Design review of the part built by this model. Coordinates are the model's own, in mm. A direction names the side the tool comes from. Coordinates: 2 decimals unless noted, no trailing zeros. Write each loop counter-clockwise with the first axis right and the second up, starting at its lowest first coordinate (ties: lowest second). Pieces come first, ordered by that corner, then holes.
Autodesk Inventor part; units mm, degrees
ref_plane "YZ Plane" through (0, 0, 0) normal (1, 0, 0) x (0, 1, 0)
ref_plane "XZ Plane" through (0, 0, 0) normal (0, 1, 0) x (-1, 0, 0)
ref_plane "XY Plane" through (0, 0, 0) normal (0, 0, 1) x (1, 0, 0)
sketch "Sketch1" plane through (0, 0, 0) normal (0, 1, 0) x (-1, 0, 0)
  line L0 (-60, 75) -> (60, 75)
  line L1 (60, -75) -> (-60, -75)
  line L2 (-60, 75) -> (60, -75) construction
  line L3 (60, 75) -> (-60, -75) construction
  line L4 (-60, -75) -> (-60, -55)
  line L5 (-60, -55) -> (-57, -55)
  line L6 (-60, -55) -> (-57, -55)
  line L7 (-57, -55) -> (-57, -42.5)
  line L8 (-57, -42.5) -> (-60, -42.5)
  line L9 (-60, -42.5) -> (-60, -55)
  line L10 (-57, -42.5) -> (-38.1, -42.5)
  line L11 (-38.1, -42.5) -> (-35.1, -42.5)
  line L12 (-35.1, -42.5) -> (-35.1, -55)
  line L13 (-35.1, -55) -> (-38.1, -55)
  line L14 (-38.1, -55) -> (-38.1, -42.5)
  line L15 (0, 75) -> (0, 64.8)
  line L16 (0, 64.8) -> (-33, 64.8)
  line L17 (-33, 64.8) -> (33, 64.8)
  circle A0 centre (-33, 64.8) radius 1.4
  circle A1 centre (33, 64.8) radius 1.4
  line L18 (0, 75) -> (0, 40)
  line L19 (0, 40) -> (-20, 40)
  line L20 (-20, 40) -> (20, 40)
  circle A2 centre (20, 40) radius 1.4
  circle A3 centre (-20, 40) radius 1.4
  line L21 (-60, -75) -> (-60, -5)
  line L22 (-4, -5) -> (4, -5)
  line L23 (-60, 75) -> (-60, 60)
  line L24 (-60, 60) -> (60, 60)
  line L25 (-20, 40) -> (-21.4, 40)
  line L26 (20, 40) -> (21.4, 40)
  line L27 (-30, 40) -> (-30, 10)
  line L28 (-30, 10) -> (-60, 0)
  line L29 (30, 40) -> (30, 10)
  line L30 (30, 10) -> (60, -5)
  line L31 (-30, 40) -> (-30, 48)
  line L32 (-30, 48) -> (-60, 60)
  line L33 (30, 40) -> (30, 48)
  line L34 (30, 48) -> (60, 60)
  line L35 (0, 75) -> (0, -75)
  line L36 (0, -75) -> (-60, -75)
  line L37 (0, 75) -> (-60, 75)
  line L38 (60, -70) -> (60, -55)
  line L39 (60, -55) -> (57, -55)
  line L40 (57, -55) -> (57, -42.5)
  line L41 (57, -42.5) -> (60, -42.5)
  line L42 (60, -42.5) -> (60, -55)
  line L43 (57, -42.5) -> (38.1, -42.5)
  line L44 (38.1, -42.5) -> (35.1, -42.5)
  line L45 (35.1, -42.5) -> (35.1, -55)
  line L46 (35.1, -55) -> (38.1, -55)
  line L47 (38.1, -55) -> (38.1, -42.5)
  line L48 (60, 75) -> (52, 75)
  line L49 (52, 75) -> (52, 70)
  line L50 (52, 70) -> (60, 70)
  line L51 (60, 70) -> (60, 75)
  line L52 (-60, 75) -> (-52, 75)
  line L53 (-52, 75) -> (-52, 70)
  line L54 (-52, 70) -> (-60, 70)
  line L55 (-60, 70) -> (-60, 75)
  line L56 (60, 70) -> (52, 75)
  line L57 (-52, 75) -> (-60, 70)
  line L58 (60, 75) -> (60, 60)
  line L59 (60, -5) -> (60, -70)
  line L60 (-60, -75) -> (-60, 0)
  line L61 (-60, 60) -> (-60, 75)
  line L62 (57, -75) -> (50, -75)
  line L63 (50, -75) -> (50, -70)
  line L64 (50, -70) -> (60, -70)
  line L65 (60, -70) -> (60, -75)
  line L66 (-60, -75) -> (-50, -75)
  line L67 (-50, -75) -> (-50, -70)
  line L68 (-50, -70) -> (-60, -70)
  line L69 (-60, -70) -> (-60, -75)
  line L70 (-60, -70) -> (-50, -75)
  line L71 (60, -70) -> (50, -75)
  line L72 (33, 64.8) -> (33, 62.8)
  line L73 (33, 62.8) -> (-33, 62.8)
  line L74 (-33, 62.8) -> (-33, 64.8)
  line L75 (0, 62.8) -> (10, 62.8)
  line L76 (10, 62.8) -> (-10, 62.8)
  line L77 (-10, 61.05) -> (10, 61.05)
  line L78 (10, 61.05) -> (10, 64.55)
  line L79 (10, 64.55) -> (-10, 64.55)
  line L80 (-10, 64.55) -> (-10, 61.05)
  line L81 (-10, 61.05) -> (10, 64.55) construction
  line L82 (10, 61.05) -> (-10, 64.55) construction
  line L83 (10, 61.05) -> (-10, 61.05)
  line L84 (-10, 61.05) -> (-10, 60)
  line L85 (-10, 60) -> (10, 60)
  line L86 (10, 60) -> (10, 61.05)
  line L87 (30, 48) -> (30, 23)
  line L88 (30, 23) -> (60, -5)
  line L89 (-30, 48) -> (-30, 23)
  line L90 (-30, 23) -> (-60, 0)
  line L91 (60, -75) -> (31, -75)
  line L92 (31, -75) -> (31, -67)
  line L93 (31, -67) -> (60, -67)
  line L94 (60, -67) -> (60, -75)
  line L95 (-60, -75) -> (-31, -75)
  line L96 (-31, -75) -> (-31, -67)
  line L97 (-31, -67) -> (-60, -67)
  line L98 (-60, -67) -> (-60, -75)
  circle A4 centre (-31, -67) radius 1.4
  circle A5 centre (31, -67) radius 1.4
  point P0 (0, 0)
  dimension "d16" = 2.8
  dimension "d17" = 2.8
  dimension "d0" = 120
  dimension "d1" = 150
  dimension "d2" = 20
  dimension "d3" = 3
  dimension "d4" = 3
  dimension "d5" = 12.5
  dimension "d6" = 18.9
  dimension "d7" = 3
  dimension "d8" = 10.2
  dimension "d9" = 33
  dimension "d10" = 66
  dimension "d11" = 2.8
  dimension "d12" = 2.8
  dimension "d13" = 35
  dimension "d14" = 20
  dimension "d15" = 40
  dimension "d18" = 70
  dimension "d19" = 15
  dimension "d20" = 10
  dimension "d21" = 10
  dimension "d22" = 30
  dimension "d23" = 30
  dimension "d24" = 8
  dimension "d25" = 8
  dimension "d26" = 20
  dimension "d27" = 3
  dimension "d28" = 12.5
  dimension "d29" = 18.9
  dimension "d30" = 3
  dimension "d31" = 8
  dimension "d32" = 5
  dimension "d33" = 8
  dimension "d34" = 5
  dimension "d35" = 10
  dimension "d36" = 5
  dimension "d37" = 10
  dimension "d38" = 5
  dimension "d42" = 2
  dimension "d43" = 10
  dimension "d44" = 20
  dimension "d45" = 3.5
  dimension "d47" = 25
  dimension "d48" = 25
  dimension "d49" = 29
  dimension "d50" = 8
  dimension "d51" = 29
  dimension "d52" = 8
  dimension "d53" = 2.8
  dimension "d54" = 2.8
extrude "Extrusion1" add sketch "Sketch1" along normal blind 5 contours L0 L15 L16 A0 L74 L73 L80 L84 L24 L23 L54 L53 | L53 L54 L57 | L0 L49 L50 L58 L24 L86 L78 L73 L72 A1 L17 L15 | L24 L18 L35 L1 L96 A4 L97 L4 L5 L7 L8 L21 L60 L28 L27 L31 L32 | L56 L50 L49 | L18 L79 L80 L73 L74 A0 L16 | L17 A1 L72 L73 L78 L79 L18 | L24 L34 L33 L29 L30 L59 L41 L40 L39 L38 L93 A5 L92 L1 L35 L18 | L27 L28 L90 | L88 L30 L29 | L92 A5 L93 L38 L64 L63 L1 | L1 L67 L68 L4 L97 A4 L96 | L63 L64 L71 | L70 L68 L67
fillet "Fillet1" radius 3 14 edges at (-52, 2.5, 75) (-60, 2.5, 70) (-60, 2.5, 60) (-30, 2.5, 48) (-60, 2.5, -5) (-50, 2.5, -75) (-60, 2.5, -70) (60, 2.5, -70) (50, 2.5, -75) (60, 2.5, 0) (30, 2.5, 48) (52, 2.5, 75) (60, 2.5, 70) (60, 2.5, 60)
fillet "Fillet2" radius 1 4 edges at (-10, 2.5, 64.55) (-10, 2.5, 60) (10, 2.5, 64.55) (10, 2.5, 60)
properties part number "KhungDuoi"
(1) Mouldability with a two-part tool opening along Z and no side actions: class faces 1 (the flat face through (60, 2, -62)), 2 (the flat face through (57, 2, -49)), 3 (the flat face through (55.619, 2.465, 72.738)), 4 (the flat face through (38.1, 2, -49)) as +Z half, -Z half, draft (parallel to the pull), parting line (faces both ways), or undercut.
(2) Consider section A-A (x = -41). Give the boundary of the cut face in (y, z).
(3) Insertion check: pin 1 Ø3 at (x, z) = (33, 64.8) entering from -Y; pin 2 Ø2 at (x, z) = (-33, 64.8) entering from -Y; pin 3 Ø2.5 at (x, y) = (59, 3.5) entering from +Z; pin 4 Ø1.5 at (y, z) = (2, -51.5) entering from +X. Each pin has a flat end and moves straight along its axis. Give the tip position at first contact, or say it passes through.
(4) Consider section C-C (z = 29). Give the boundary of the cut face in (x, y), plus the area to 3 significant figures.
(5) Wall thickness on line 1 (X direction, y = 3.8, z = 64.8); line 2 (X direction, y = 1.4, z = 40); line 3 (Z direction, x = -33, y = 1.45): over which ranges is each line inside the solid? List them lowest first.
(6) Consider section D-D (z = 10.5). Give the boundary of the cut face in (x, y).
(7) For faces 5 (the flat face through (-59, 2, -55)), 6 (the flat face through (35.1, 2, -49)), 7 (the flat face through (58, 2, -42.5)), list the 3-axis set-ups (+Z, -Z, +X, -X, +Y, -Y) from which the entire face can be reached by the end or side of a thin tool; tool diameter is ignored.
(8) Consider section B-B (y = 4.1). State how many separate pieces and enclosed holes the cut face has, plus the area to 3 significant figures.
Results:
1. face 1: draft
1. face 2: undercut
1. face 3: +Z half
1. face 4: undercut
2. outline: (0, -75) - (5, -75) - (5, 12.73) - (0, 12.73) - close; (0, 52.4) - (5, 52.4) - (5, 75) - (0, 75) - close
3. pin 1: stops at y = 0
3. pin 2: passes through
3. pin 3: stops at z = 71.41
3. pin 4: stops at x = 57
4. outline: (-30, 0) - (30, 0) - (30, 5) - (-30, 5) - close
4. area: 300 mm2
5. line 1: x = -60 to -34.4, -31.6 to 31.6, 34.4 to 60
5. line 2: x = -30 to -21.4, -18.6 to 18.6, 21.4 to 30
5. line 3: z = -75 to 20.2, 49.2 to 63.4, 66.2 to 75
6. outline: (-43.39, 0) - (46.3, 0) - (46.3, 5) - (-43.39, 5) - close
7. face 5: -X, +Y, -Y
7. face 6: +Y, -Y
7. face 7: +X, +Y, -Y
8. separate pieces: 1
8. enclosed holes: 9
8. area: 15,000 mm2
